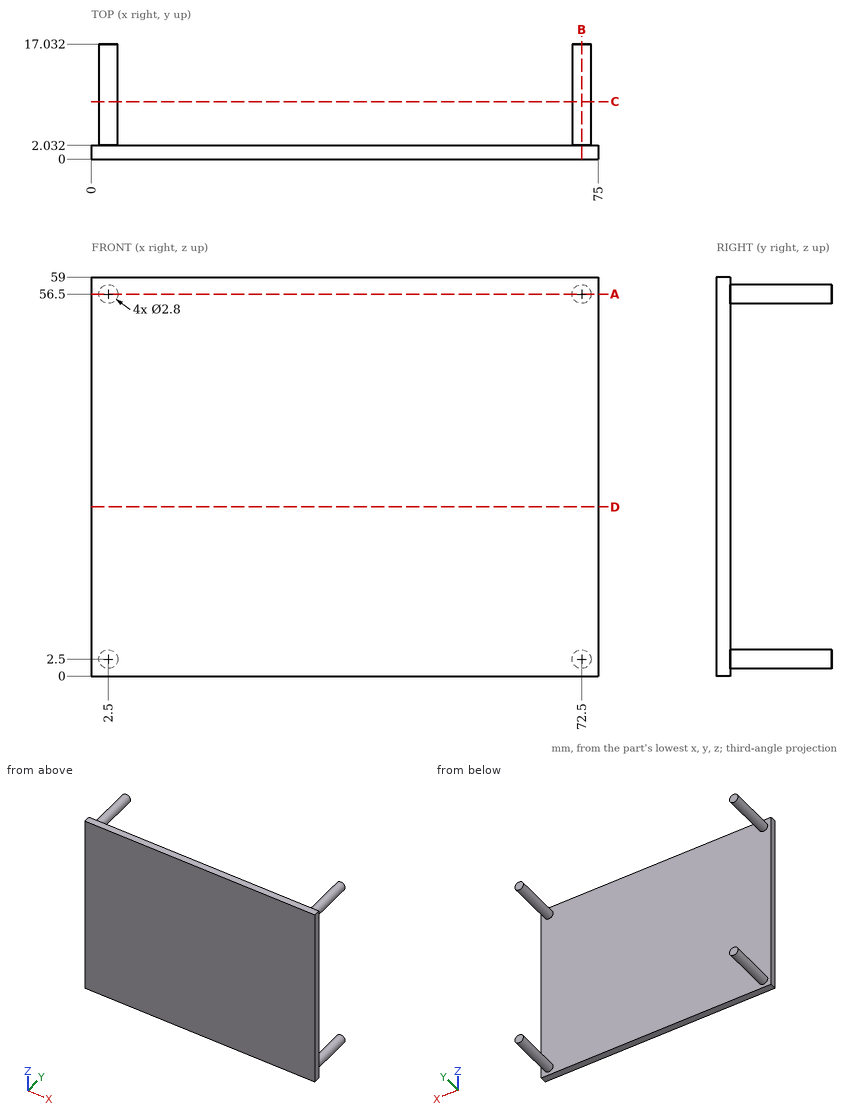
Could you check a few things on this drawing? It's one solid part, dimensions in mm from its lowest x, y, z. Coordinates: 2 decimals unless noted, no trailing zeros. Order: outer loops, then holes, each group sorted by start corner. A loop starts at its lowest first (then second) coordinate and runs counter-clockwise, first axis right, second up. Notation, with made-up numbers: (20, -27.5) - (40, -27.5) arc R30 ccw to (40, 6.5) - close; hole circle Ø8 at (61.25, 77). An arc over 180 degrees is marked (long way). One line per question, with ' | ' between items. Start each with the question number.
1. If we section it at D-D (z = 25): Write out the boundary of the cut face in (x, y).
2. If we section it at A-A (z = 56.5): Write out the boundary of the cut face in (x, y), and give its area (3 significant figures).
3. If we section it at C-C (y = 8.5): Write out the boundary of the cut face in (x, z), and give its area (3 significant figures).
4. If we section it at B-B (x = 72.5): Write out the boundary of the cut face in (y, z), and give its area (3 significant figures).
5. I'm going to push flat-ended pins straight in: pin 1 Ø10 at (x, z) = (33, 51) entering from +Y; pin 2 Ø1.5 at (x, z) = (59.5, 21) entering from -Y. Where does each tip first touch, or does it pass through?
6. Please list where this line runs through material, in increasing order: line 1 along Y through (x, z) = (58, 9.5). Write a range as [from, to].
Model answer:
1) outline: (0, 0) - (75, 0) - (75, 2.03) - (0, 2.03) - close
2) outline: (0, 0) - (75, 0) - (75, 2.03) - (73.9, 2.03) - (73.9, 17.03) - (71.1, 17.03) - (71.1, 2.03) - (3.9, 2.03) - (3.9, 17.03) - (1.1, 17.03) - (1.1, 2.03) - (0, 2.03) - close | area: 236 mm²
3) outline: circle Ø2.8 at (2.5, 2.5); circle Ø2.8 at (2.5, 56.5); circle Ø2.8 at (72.5, 2.5); circle Ø2.8 at (72.5, 56.5) | area: 24.6 mm²
4) outline: (0, 0) - (2.03, 0) - (2.03, 1.1) - (17.03, 1.1) - (17.03, 3.9) - (2.03, 3.9) - (2.03, 55.1) - (17.03, 55.1) - (17.03, 57.9) - (2.03, 57.9) - (2.03, 59) - (0, 59) - close | area: 204 mm²
5) pin 1: stops at y = 2.03 | pin 2: stops at y = 0
6) line 1: y = [0, 2.03]
